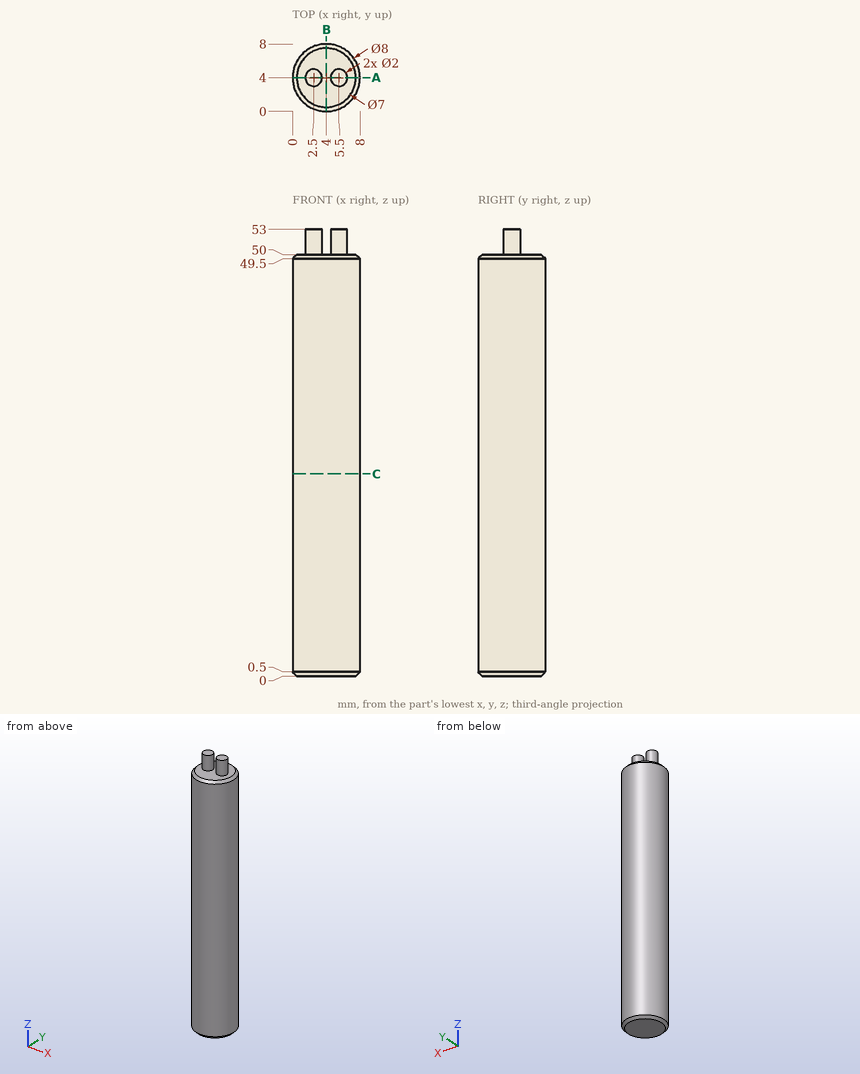
Source: three-view drawing plus pictorial views. Frame: mm from the lowest corner of the part. Give positions to 0.01 mm unless a question says otherwise; leave off trailing zeros. Order: outer loops, then holes, each group sorted by start corner. A loop starts at its lowest first (then second) coordinate and runs counter-clockwise, first axis right, second up. Notation, with made-up numbers: M 22,-23.5 L 41,-23.5 A25 ccw 41,-3.5 Z; hole C 30.5,-27 d11. An arc over 180 degrees is marked long. One line per question, with ' | ' between items.
1) Contact query for flat-ended pins moving along their axis: P1, Ø1, axis at x = 2, z = 13.5, coming from the -Y side; P2, Ø1.5, axis at x = 1.5, z = 6.5, coming from the +Y side. Output: stop coordinate, or through.
Filled in:
P1: stops at y = 0.29 | P2: stops at y = 7.6
2) Section A-A on y = 4. Output: boundary loops of the cut face in (x, z), and give its area (4 significant figures).
Filled in:
outline: M 0,0.5 L 0.5,0 L 7.5,0 L 8,0.5 L 8,49.5 L 7.5,50 L 6.5,50 L 6.5,53 L 4.5,53 L 4.5,50 L 3.5,50 L 3.5,53 L 1.5,53 L 1.5,50 L 0.5,50 L 0,49.5 Z | area: 411.5 mm2
3) Section C-C on z = 24. Output: boundary loops of the cut face in (x, y), and give its area (3 significant figures).
Filled in:
outline: C 4,4 d8 | area: 50.3 mm2
4) Section B-B on x = 4. Output: boundary loops of the cut face in (y, z), and give its area (4 significant figures).
Filled in:
outline: M 0,0.5 L 0.5,0 L 7.5,0 L 8,0.5 L 8,49.5 L 7.5,50 L 0.5,50 L 0,49.5 Z | area: 399.5 mm2
5) Ray query, L1, parallel to Z at x = 1.75, y = 2.75; L2, parallel to Y at x = 4.25, z = 32.5; L3, parallel to Y at x = 5.75, z = 14.5. Return the intervals inside material, ascending.
Filled in:
L1: z = 0 to 50 | L2: y = 0.01 to 7.99 | L3: y = 0.4 to 7.6
